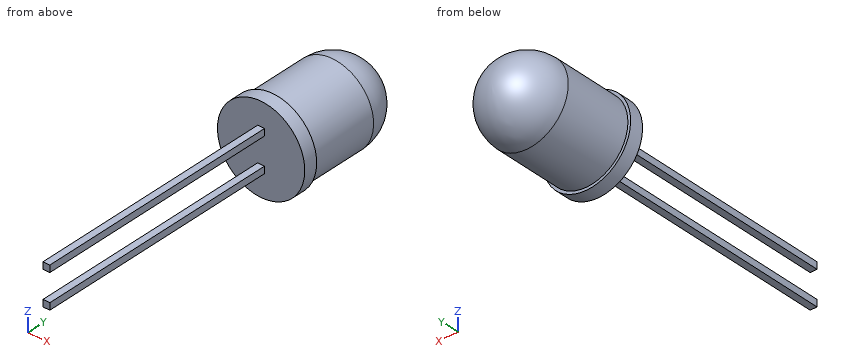
from build123d import *

# Parameters (mm, degrees)
SKETCH2_R           = 3.2
BOSS_EXTRUDE1_DEPTH = 1
SKETCH3_W           = 0.5
SKETCH3_H           = 0.5
BOSS_EXTRUDE2_DEPTH = 18


with BuildPart() as part:
    # Sketch1 → Revolve1 (revolve)
    with BuildSketch(Plane.XY, mode=Mode.PRIVATE) as revolve1_sk:
        with BuildLine():
            Line((0, 5), (0, 8))
            ThreePointArc((0, 8), (-2.121320344, 7.121320344), (-3, 5))
            Line((-3, 5), (-3, 0))
            Line((-3, 0), (0, 0))
            Line((0, 0), (0, 5))
        make_face()
    revolve(revolve1_sk.sketch.rotate(Axis((0, 0, 0), (0, 1, 0)), 270), axis=Axis((0, 0, 0), (0, 1, 0)))

    # Sketch2 → Boss-Extrude1 (add)
    with BuildSketch(Plane(origin=(0, 0, 0), x_dir=(-1, 0, 0), z_dir=(0, -1, 0))):
        with Locations(Location((0, 0, 0), (0, 0, 90))):
            Circle(SKETCH2_R)
    extrude(amount=BOSS_EXTRUDE1_DEPTH)

    # Sketch3 → Boss-Extrude2 (add)
    with BuildSketch(Plane(origin=(0, -1, 0), x_dir=(-1, 0, 0), z_dir=(0, -1, 0))):
        with Locations((0, -1.25)):
            Rectangle(SKETCH3_W, SKETCH3_H)
    boss_extrude2 = extrude(amount=BOSS_EXTRUDE2_DEPTH)

    # Mirror1: Boss-Extrude2 across plane
    add(boss_extrude2.mirror(Plane.XY))


solid = part.part
Could you check a few things on this model? Use its own coordinates, in mm. Coordinates: 2 decimals unless noted, no trailing zeros. Write each loop counter-clockwise with the first axis right and the second up, starting at its lowest first coordinate (ties: lowest second). Pieces come first, ordered by that corner, then holes. Notation, with made-up numbers: (79.25, -34) - (83.25, -34) arc R28 ccw to (83.25, -9) - close; hole circle Ø10 at (63, 10.25). An arc over 180 degrees is marked (long way). Write item = value, one per line.
1) Suppose I cut it at C-C on x = 0. Please give me the cut outline in (y, z).
Result set:
outline = (-19, -1.5) - (-1, -1.5) - (-1, -3.2) - (0, -3.2) - (0, -3) - (5, -3) arc R3 ccw to (5, 3) - (0, 3) - (0, 3.2) - (-1, 3.2) - (-1, 1.5) - (-19, 1.5) - (-19, 1) - (-1, 1) - (-1, -1) - (-19, -1) - close
2) Will these pins go through, and if not, where does the flat tip stop? pin 1 Ø1.5 at (x, z) = (-1, 0) entering from +Y; pin 2 Ø1 at (x, z) = (-2, -1.5) entering from -Y; pin 3 Ø2 at (x, z) = (2.5, -2) entering from +Y.
Result set:
pin_1 = 7.99
pin_2 = -1
pin_3 = 7.04
3) Suppose I cut it at A-A on y = -14.5. Please give me the cut outline in (x, z), plus the area to 3 significant figures.
Result set:
outline = (-0.25, -1.5) - (0.25, -1.5) - (0.25, -1) - (-0.25, -1) - close; (-0.25, 1) - (0.25, 1) - (0.25, 1.5) - (-0.25, 1.5) - close
area = 0.500 mm2
4) Please list where these lines run through material, in increasing order: line 1 (Y direction, x = 2, z = -1.75); line 2 (X direction, y = 1.5, z = -1.5); line 3 (X direction, y = 4.5, z = 0.5). Write a range as [from, to].
Result set:
line_1 = [-1, 6.39]
line_2 = [-2.6, 2.6]
line_3 = [-2.96, 2.96]
5) Suppose I cut it at B-B on z = -2.25. Please give me the cut outline in (x, y), plus the area to 3 significant figures.
Result set:
outline = (-2.28, -1) - (2.28, -1) - (2.28, 0) - (1.98, 0) - (1.98, 5) arc R1.98 ccw to (-1.98, 5) - (-1.98, 0) - (-2.28, 0) - close
area = 30.6 mm2
6) Suppose I cut it at D-D on y = -0.75. Please give me the cut outline in (x, z).
Result set:
outline = circle Ø6.4 at (0, 0)
